from build123d import *

# Parameters (mm, degrees)
F0_W     = 70
F0_H     = 35
F1_DEPTH = 50
F3_DEPTH = 23
F5_DEPTH = 11
F6_W     = 14
F6_H     = 18
F7_DEPTH = 6
F8_W     = 20
F8_H     = 8
F9_DEPTH = 25


with BuildPart() as f1:
    # F0 (on Front) → F1 (new body)
    with BuildSketch(Plane.XZ):
        with Locations((1.583831, 6.053839)):
            Rectangle(F0_W, F0_H)
    extrude(amount=-F1_DEPTH)

    # F2 (on face) → F3 (cut)
    with BuildSketch(Plane.XY.offset(23.553839)):
        Polygon((-19.416169, 0), (36.583831, 0), (36.583831, 20), (28.583831, 20), (28.583831, 36), (-19.416169, 36), align=None)
    extrude(amount=-F3_DEPTH, mode=Mode.SUBTRACT)

    # F4 (on face) → F5 (cut)
    with BuildSketch(Plane.XY.offset(23.553839)):
        Polygon((16.583831, 36), (28.583831, 36), (28.583831, 20), (36.583831, 20), (36.583831, 50), (16.583831, 50), align=None)
    extrude(amount=-F5_DEPTH, mode=Mode.SUBTRACT)

    # F6 (on face) → F7 (cut)
    with BuildSketch(Plane.XY.offset(23.553839)):
        with Locations((-26.416169, 26)):
            Rectangle(F6_W, F6_H)
    extrude(amount=-F7_DEPTH, mode=Mode.SUBTRACT)

    # F8 (on face) → F9 (cut)
    with BuildSketch(Plane.XY.offset(0.553839)):
        with Locations((8.583831, 4)):
            Rectangle(F8_W, F8_H)
    extrude(amount=-F9_DEPTH, mode=Mode.SUBTRACT)


solid = f1.part
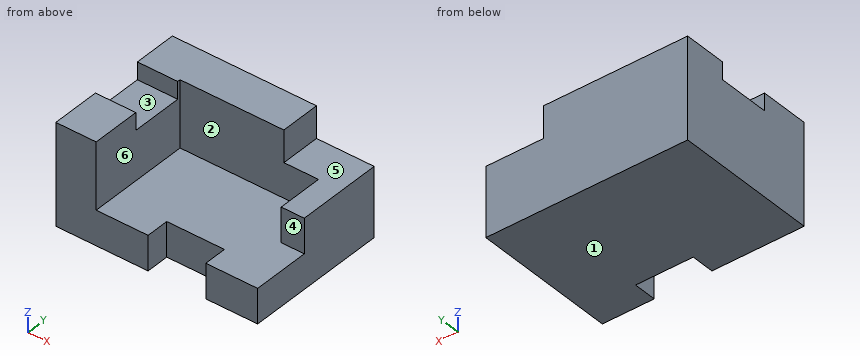
Geometry: final body of the model. Coordinates: model frame, mm. Face numbers are marked on the shaded views. A direction names the side the tool comes from. Coordinates: 2 decimals unless noted, no trailing zeros. Loops run counter-clockwise (first coordinate to the right, second up) from the corner with the lowest first, then second, coordinate; pieces in that order, holes last. Notation, with made-up numbers: (-5, -9.5) - (44, -9.5) arc R20 cw to (44, 16.5) - close; hole circle Ø7 at (45, -11.5). An arc over 180 degrees is marked (long way). Put each result on its own line as item: value. Start each with the question number.
Q1. Pin query (flat end, axial travel): pin 1 Ø5 at (x, y) = (27, 36.5) entering from +Z; pin 2 Ø1.8 at (x, z) = (-26, 20.5) entering from -Y; pin 3 Ø6.5 at (x, z) = (33.5, 7.5) entering from -Y; pin 4 Ø7 at (x, z) = (4, 6.5) entering from -Y. Return the tip coordinate at first contact, or that it passes through.
Q2. Cut plane D-D, the plane y = 28.5. Return loops of the section in (x, z), and give its area (3 significant figures).
Q3. Line query: line 1 (Y direction, x = -9, z = 14); line 2 (X direction, y = 25, z = 1); line 3 (Z direction, x = -15.5, y = 9.5). Output: solid intervals per line, ascending.
Q4. Cut plane A-A, the plane z = 19.5. Return loops of the section in (x, y).
Q5. Cut plane B-B, the plane y = 5. Return loops of the section in (x, z), and give its area (3 significant figures).
Q6. Cut plane C-C, the plane x = -23. Return loops of the section in (y, z), and give its area (3 significant figures).
Q7. Pull-direction query (Y, two-part tool) for the marked faces 1, 2 and 3; classes: released by +Y, released by -Y, zero draft, split by the parting line, or undercut.
Q8. Set-up query: the marked faces 4, 5 and 6. Return all of +Z, -Z, +X, -X, +Y, -Y with unobstructed straight access to the full face (end or side cutting, diameter ignored); none if empty.
Filled sheet:
1. pin 1: z = 12.55
1. pin 2: y = 0
1. pin 3: y = 20
1. pin 4: y = 36
2. outline: (-33.42, -11.45) - (36.58, -11.45) - (36.58, 12.55) - (28.58, 12.55) - (28.58, 0.55) - (-19.42, 0.55) - (-19.42, 17.55) - (-33.42, 17.55) - close
2. area: 1,170 mm²
3. line 1: 36 to 50
3. line 2: -33.42 to -19.42, 28.58 to 36.58
3. line 3: -11.45 to 0.55
4. outline: (-33.42, 0) - (-19.42, 0) - (-19.42, 17) - (-33.42, 17) - close; (-33.42, 35) - (-19.42, 35) - (-19.42, 36) - (16.58, 36) - (16.58, 50) - (-33.42, 50) - close
5. outline: (-33.42, -11.45) - (-1.42, -11.45) - (-1.42, 0.55) - (-19.42, 0.55) - (-19.42, 23.55) - (-33.42, 23.55) - close; (18.58, -11.45) - (36.58, -11.45) - (36.58, 0.55) - (18.58, 0.55) - close
5. area: 922 mm²
6. outline: (0, -11.45) - (50, -11.45) - (50, 23.55) - (35, 23.55) - (35, 17.55) - (17, 17.55) - (17, 23.55) - (0, 23.55) - close
6. area: 1,640 mm²
7. face 1: zero draft
7. face 2: released by -Y
7. face 3: undercut
8. face 4: +Z, +X, -Y
8. face 5: +Z, +X, +Y, -Y
8. face 6: +Z, -Y
